from build123d import *

# Parameters (mm, degrees)
F0_R     = 1.25
F1_DEPTH = 9
F2_SIZE  = 0.3
F3_R     = 0.7
F4_DEPTH = 0.5
F4_TAPER = 20


# Not quite as in the source:
# - a pattern or mirror of a feature is missing from the dataset's text; its kind, count and spacing are read off the source's solid


with BuildPart() as f1:
    # F0 (on Right) → F1 (new body, symmetric)
    with BuildSketch(Plane.YZ):
        Circle(F0_R)
    extrude(amount=F1_DEPTH, both=True)

    # F2
    f2_edges = [f1.edges().sort_by_distance(p)[0] for p in [
        (-9, -1.25, 0),
        (9, -1.25, 0),
    ]]
    chamfer(f2_edges, length=F2_SIZE)

    # F3 (on face) → F4 (cut)
    with BuildSketch(Plane(origin=(-9, 0, 0), x_dir=(0, -1, 0), z_dir=(-1, 0, 0))):
        Circle(F3_R)
    f4 = extrude(amount=-F4_DEPTH, taper=F4_TAPER, mode=Mode.SUBTRACT)

    # F4_copies: F4 across plane
    add(f4.mirror(Plane(origin=(0, 0, 0), x_dir=(0, 0, 1), z_dir=(1, 0, 0))), mode=Mode.SUBTRACT)


solid = f1.part
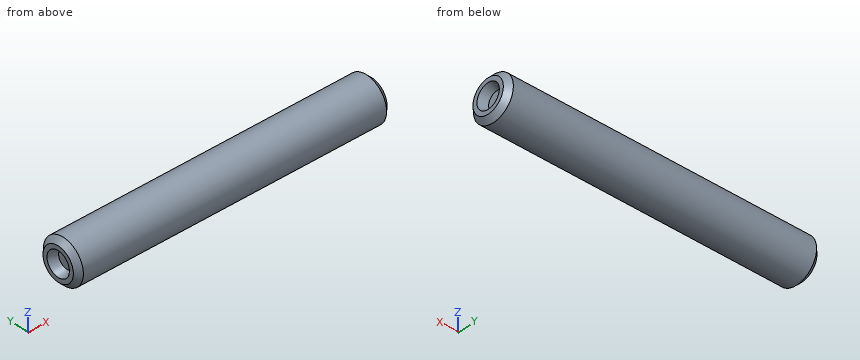
Read the model definition and answer for the solid it produces. Units are mm, in the model's axes. Give positions to 0.01 mm unless a question says otherwise; leave off trailing zeros. Write each loop counter-clockwise with the first axis right and the second up, starting at its lowest first coordinate (ties: lowest second). Pieces come first, ordered by that corner, then holes. Notation, with made-up numbers: (-10.75, -17.5) - (24.25, -17.5) arc R16 cw to (24.25, -7.5) - close; hole circle Ø8 at (4, -18). An arc over 180 degrees is marked (long way). Return JSON: item names as keys, results as strings.
Q1. Consider line 1 along X through (y, z) = (0.25, 0); line 2 along Y through (x, z) = (-4, 0.1). Determine where each line is inside the solid, lowest interval first. Write a range as [from, to].
Reply:
{"line 1": "[-8.5, 8.5]", "line 2": "[-1.25, 1.25]"}
Q2. A cutting plane is placed at A-A, the plane y = 0. Determine the outline of the cut face in (x, z).
Reply:
{"outline": "(-9, -0.95) - (-8.7, -1.25) - (8.7, -1.25) - (9, -0.95) - (9, -0.7) - (8.5, -0.52) - (8.5, 0.52) - (9, 0.7) - (9, 0.95) - (8.7, 1.25) - (-8.7, 1.25) - (-9, 0.95) - (-9, 0.7) - (-8.5, 0.52) - (-8.5, -0.52) - (-9, -0.7) - close"}
Q3. A cutting plane is placed at B-B, the plane x = -4.5. Determine the outline of the cut face in (y, z).
Reply:
{"outline": "circle Ø2.5 at (0, 0)"}
